Part model, mm, in its own coordinate system. Face numbers are marked on the shaded views. Round coordinates to 2 decimals unless told otherwise and drop trailing zeros. Loops run counter-clockwise (first coordinate to the right, second up) from the corner with the lowest first, then second, coordinate; pieces in that order, holes last.
from build123d import *

# Parameters (mm, degrees)
F0_W     = 86.36
F0_H     = 25.4
F0_R     = 12.2809
F1_DEPTH = 25.4


with BuildPart() as f1:
    # F0 (on Front) → F1 (new body)
    with BuildSketch(Plane.XZ):
        with BuildLine():
            ThreePointArc((24.946787, 31.153673), (25.410052, 28.376437), (25.5651, 25.5651))
            ThreePointArc((25.5651, 25.5651), (-2.811337, 0.155048), (-24.946787, 31.153673))
            Line((-24.946787, 31.153673), (-43.18, -16.261408))
            Line((-43.18, -16.261408), (43.18, -16.261408))
            Line((43.18, -16.261408), (24.946787, 31.153673))
        make_face()
        with Locations((0, -28.961408)):
            Rectangle(F0_W, F0_H)
        with BuildLine():
            ThreePointArc((-24.946787, 31.153673), (-2.811337, 0.155048), (25.5651, 25.5651))
            ThreePointArc((25.5651, 25.5651), (25.410052, 28.376437), (24.946787, 31.153673))
            ThreePointArc((24.946787, 31.153673), (0, 51.1302), (-24.946787, 31.153673))
        make_face()
        with Locations((0, 25.5651)):
            Circle(F0_R, mode=Mode.SUBTRACT)
    extrude(amount=F1_DEPTH)


solid = f1.part
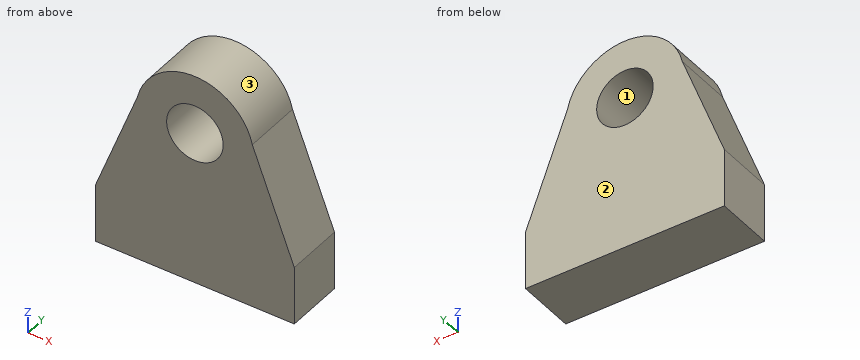
1) Wall check: line 1 along Z through (x, y) = (0, -11.5); line 2 along X through (y, z) = (-21.5, 20); line 3 along X through (y, z) = (-21, 35.5). Give the ranges that are in metal, low to high.
Values:
line 1: z = -41.66 to 13.28, 37.85 to 51.13
line 2: x = -29.24 to -10.95, 10.95 to 29.24
line 3: x = -23.56 to -7.22, 7.22 to 23.56
2) Slice it at B-B, the plane z = 16. Give the cut face in (x, y).
Values:
outline: (-30.77, -25.4) - (-7.7, -25.4) - (-7.7, 0) - (-30.77, 0) - close; (7.7, -25.4) - (30.77, -25.4) - (30.77, 0) - (7.7, 0) - close
3) Mould opens along Z. For the marked faces 1, 2 and 3 say: released by +Z, released by -Z, zero draft, split by the parting line, or undercut.
Values:
face 1: undercut
face 2: zero draft
face 3: released by +Z
4) Slice it at A-A, the plane x = 0. Give the cut face in (y, z).
Values:
outline: (-25.4, -41.66) - (0, -41.66) - (0, 13.28) - (-25.4, 13.28) - close; (-25.4, 37.85) - (0, 37.85) - (0, 51.13) - (-25.4, 51.13) - close
5) Slice it at D-D, the plane z = 43. Give the cut face in (x, y).
Values:
outline: (-18.7, -25.4) - (18.7, -25.4) - (18.7, 0) - (-18.7, 0) - close
6) Drop flat-ended pins along their axis: pin 1 Ø3 at (y, z) = (-17, 39.5) entering from -X; pin 2 Ø4 at (y, z) = (-6.5, -3.5) entering from -X. Give the stop position or say it passes through.
Values:
pin 1: stops at x = -22.34
pin 2: stops at x = -39.04
7) Slice it at C-C, the plane y = -3. Give the cut face in (x, z).
Values:
outline: (-43.18, -41.66) - (43.18, -41.66) - (43.18, -16.26) - (24.95, 31.15) arc R25.57 ccw to (-24.95, 31.15) - (-43.18, -16.26) - close; hole circle Ø24.56 at (0, 25.57)
